For this review, take the finished solid that the model builds, in its own axes (mm). A direction names the side the tool comes from. Give positions to 0.01 mm unless a question says otherwise; leave off trailing zeros. Order: outer loops, then holes, each group sorted by start corner. A loop starts at its lowest first (then second) coordinate and runs counter-clockwise, first axis right, second up. Notation, with made-up numbers: (1, 78) - (48, 78) arc R18 cw to (48, 84) - close; hole circle Ø6 at (43, 24). An arc over 180 degrees is marked (long way). Put each result on its own line as item: value. Start each with the question number.
```python
from build123d import *

# Parameters (mm, degrees)
SKETCH1_R           = 8
SKETCH1_W           = 5
SKETCH1_H           = 10
BOSS_EXTRUDE1_DEPTH = 5
SKETCH2_R           = 2
CUT_EXTRUDE1_DEPTH  = 15
CIRPATTERN1_COUNT   = 3


with BuildPart() as part:
    # Sketch1 → Boss-Extrude1 (new, symmetric)
    # profile 1 of 7: a face of its own
    with BuildSketch(Plane(origin=(0, 0, 0), x_dir=(1, 0, 0), z_dir=(0, 1, 0))):
        Polygon((25, 0), (12.5, 21.650635095), (-12.5, 21.650635095), (-25, 0), (-12.5, -21.650635095), (12.5, -21.650635095), align=None)
        with Locations(Location((0, 0, 0), (0, 0, 270))):
            Circle(SKETCH1_R, mode=Mode.SUBTRACT)
    # profile 2 of 7: a face of its own
    with BuildSketch(Plane(origin=(0, 0, 0), x_dir=(1, 0, 0), z_dir=(0, 1, 0))):
        Polygon((-22.5, -4.330127019), (-25, 0), (-33.660254038, -5), (-31.160254038, -9.330127019), align=None)
    # profile 3 of 7: a face of its own
    with BuildSketch(Plane(origin=(0, 0, 0), x_dir=(1, 0, 0), z_dir=(0, 1, 0))):
        Polygon((-12.5, -21.650635095), (-15, -17.320508076), (-23.660254038, -22.320508076), (-21.160254038, -26.650635095), align=None)
    # profile 4 of 7: a face of its own
    with BuildSketch(Plane(origin=(0, 0, 0), x_dir=(1, 0, 0), z_dir=(0, 1, 0))):
        Polygon((15, -17.320508076), (12.5, -21.650635095), (21.160254038, -26.650635095), (23.660254038, -22.320508076), align=None)
    # profile 5 of 7: a face of its own
    with BuildSketch(Plane(origin=(0, 0, 0), x_dir=(1, 0, 0), z_dir=(0, 1, 0))):
        Polygon((33.660254038, -5), (25, 0), (22.5, -4.330127019), (31.160254038, -9.330127019), align=None)
    # profile 6 of 7: a face of its own
    with BuildSketch(Plane(origin=(0, 0, 0), x_dir=(1, 0, 0), z_dir=(0, 1, 0))):
        with Locations((10, 26.650635095)):
            Rectangle(SKETCH1_W, SKETCH1_H)
    # profile 7 of 7: a face of its own
    with BuildSketch(Plane(origin=(0, 0, 0), x_dir=(1, 0, 0), z_dir=(0, 1, 0))):
        with Locations((-10, 26.650635095)):
            Rectangle(SKETCH1_W, SKETCH1_H)
    extrude(amount=BOSS_EXTRUDE1_DEPTH, both=True)

    # Sketch2 → Cut-Extrude1 (cut, symmetric)
    with BuildSketch(Plane(origin=(0, 0, 0), x_dir=(0, 0, -1), z_dir=(1, 0, 0))):
        with Locations(Location((26.650635095, 0, 0), (0, 0, 180))):
            Circle(SKETCH2_R)
    cut_extrude1 = extrude(amount=CUT_EXTRUDE1_DEPTH, both=True, mode=Mode.SUBTRACT)

    # CirPattern1: Cut-Extrude1 ×3 about axis
    cirpattern1_axis = Axis((0, 5, 0), (0, -1, 0))
    for i in range(1, CIRPATTERN1_COUNT):
        add(cut_extrude1.rotate(cirpattern1_axis, i * 360 / CIRPATTERN1_COUNT), mode=Mode.SUBTRACT)


solid = part.part
```
1. The part is to be moulded in two halves that separate along X. For faces 1 (the face through (-8, -5, 4)), 2 (the face through (26.77, 2.292, 6.795)), 3 (the face through (32.39, 0.07, 7.2)), say which applies: released by +X, released by -X, zero draft, split by the parting line, or undercut.
2. Add section D-D, the plane z = -15. Give the boundary of the cut face in (x, y), then the cut area to 3 significant figures.
3. Add section B-B, the plane z = -6. Give the boundary of the cut face in (x, y).
4. Wall thickness on line 1 (X direction, y = 0.75, z = 0); line 2 (X direction, y = 1.25, z = 22.5); line 3 (X direction, y = -1.25, z = -24): over which ranges is each line inside the solid? List them lowest first. Write a range as from..to.
5. Add section C-C, the plane y = 0. Count the separate pieces of the cut face and the enclosed holes in it, then the cut area to 3 significant figures.
6. Clearance check with flat-ended pins moving along their axes: pin 1 (4 mm diameter, centred on y = 3.5, z = 19.5, fed in from -X); pin 2 (5 mm diameter, centred on y = -0.5, z = -25.5, fed in from -X); pin 3 (5 mm diameter, centred on x = 25.5, y = -1, fed in from +Z); pin 4 (21 mm diameter, centred on x = 0, z = 0, fed in from -Y). State where each tip first meets the part, or that it passes through.
7. Add section A-A, the plane y = 4.25. Give the boundary of the cut face in (x, z), then the cut area to 3 significant figures.
8. Tool access review of faces 4 (the face through (-7.5, 0, -29)), 5 (the face through (19.391, 2.292, 19.856)), 6 (the face through (18.698, 0.07, 10.916)): name each direction out of +Z, -Z, +X, -X, +Y, -Y from which nothing blocks a thin tool from reaching the whole face with its end or side.
Found:
1. face 1: zero draft
1. face 2: undercut
1. face 3: released by +X
2. outline: (-16.34, -5) - (16.34, -5) - (16.34, 5) - (-16.34, 5) - close
2. area: 327 mm^2
3. outline: (-21.54, -5) - (-5.29, -5) - (-5.29, 5) - (-21.54, 5) - close; (5.29, -5) - (21.54, -5) - (21.54, 5) - (5.29, 5) - close
4. line 1: x = -25..-8, 8..25
4. line 2: x = -23.56..-19.59, -15.98..-13.97, 13.97..15.98, 19.59..23.56
4. line 3: x = -12.5..-7.5, 7.5..12.5
5. separate pieces: 7
5. enclosed holes: 1
5. area: 1,600 mm^2
6. pin 1: stops at x = -22.24
6. pin 2: stops at x = -12.5
6. pin 3: stops at z = 23.46
6. pin 4: stops at y = -5
7. outline: (-33.66, 5) - (-25, 0) - (-12.5, -21.65) - (-12.5, -31.65) - (-7.5, -31.65) - (-7.5, -21.65) - (7.5, -21.65) - (7.5, -31.65) - (12.5, -31.65) - (12.5, -21.65) - (25, 0) - (33.66, 5) - (31.16, 9.33) - (22.5, 4.33) - (15, 17.32) - (23.66, 22.32) - (21.16, 26.65) - (12.5, 21.65) - (-12.5, 21.65) - (-21.16, 26.65) - (-23.66, 22.32) - (-15, 17.32) - (-22.5, 4.33) - (-31.16, 9.33) - close; hole circle Ø16 at (0, 0)
7. area: 1,720 mm^2
8. face 4: -Z, +Y, -Y
8. face 5: +X, +Y, -Y
8. face 6: +Y, -Y
